Autodesk Inventor part; units mm, degrees
ref_plane "YZ Plane" through (0, 0, 0) normal (1, 0, 0) x (0, 1, 0)
ref_plane "XZ Plane" through (0, 0, 0) normal (0, 1, 0) x (-1, 0, 0)
ref_plane "XY Plane" through (0, 0, 0) normal (0, 0, 1) x (1, 0, 0)
sketch "Sketch1" plane through (0, 0, 0) normal (0, 0, 1) x (1, 0, 0)
  line L0 (-9.2194, -2.0534) -> (-9.2194, -17.5534)
  line L1 (-9.2194, -17.5534) -> (-15.6194, -17.5534)
  line L2 (-15.6194, -17.5534) -> (-15.6194, -2.0534)
  line L3 (-15.6194, -2.0534) -> (-9.2194, -2.0534)
  line L4 (-9.2194, 19.4466) -> (-9.2194, 3.9466)
  line L5 (-9.2194, 3.9466) -> (-15.6194, 3.9466)
  line L6 (-15.6194, 3.9466) -> (-15.6194, 19.4466)
  line L7 (-15.6194, 19.4466) -> (-9.2194, 19.4466)
  line L8 (14.7806, 19.4466) -> (14.7806, 3.9466)
  line L9 (14.7806, 3.9466) -> (8.3806, 3.9466)
  line L10 (8.3806, 3.9466) -> (8.3806, 19.4466)
  line L11 (8.3806, 19.4466) -> (14.7806, 19.4466)
  line L12 (14.7806, -1.568) -> (14.7806, -17.068)
  line L13 (14.7806, -17.068) -> (8.3806, -17.068)
  line L14 (8.3806, -17.068) -> (8.3806, -1.568)
  line L15 (8.3806, -1.568) -> (14.7806, -1.568)
  line L16 (20.7806, -27.5534) -> (20.7806, 25.4466)
  line L17 (20.7806, 25.4466) -> (-21.6194, 25.4466)
  line L18 (-21.6194, 25.4466) -> (-21.6194, -27.5534)
  line L19 (-21.6194, -27.5534) -> (20.7806, -27.5534)
  circle A0 centre (-0.4194, 11.6966) radius 1.5
  circle A1 centre (-0.4194, -9.8034) radius 1.5
  point P0 (0, 0)
extrude "Extrusion1" add sketch "Sketch1" along normal blind 6
properties part number "spoolHolderHolder"
Geometry: final body of the model. Coordinates: model frame, mm. A direction names the side the tool comes from. Round coordinates to 2 decimals unless told otherwise and drop trailing zeros. Order: outer loops, then holes, each group sorted by start corner. A loop starts at its lowest first (then second) coordinate and runs counter-clockwise, first axis right, second up. Notation, with made-up numbers: M 14,23 L 18,23 A18 ccw 18,51 Z; hole C 76.5,45 d5. An arc over 180 degrees is marked long. Use one line per item in the form item = value. Start each with the question number.
Q1. Access query for faces 4 (the face through (-9.219, 12, 3)), 5 (the face through (-1, -1, 0)). Directions: +Z, -Z, +X, -X, +Y, -Y. A direction counts if a zero-diameter tool reaches every point of the face in a straight line with its end or side. Return the directions, or none.
Q2. Cut plane B-B (y = -14.5). Return loops of the section in (x, z).
Q3. Mould query, pull axis Y, two halves, no side actions, for faces 1 (the face through (-1, -27.553, 3)), 2 (the face through (-1, -1, 6)), 3 (the face through (-15.619, 12, 3)). Classes: +Y half, -Y half, draft (parallel to the pull), parting line (faces both ways), or undercut.
Q4. Cut plane C-C (z = 0.55). Return loops of the section in (x, y).
Q5. Material intervals for line 1 (Y direction, x = -12, z = 4.2); line 2 (Y direction, x = 9, z = 3.5); line 3 (X direction, y = 9, z = 0.85), sorted ascending. Write a range as [from, to].
Q6. Pin query (flat end, axial travel): pin 1 Ø2.5 at (x, y) = (-0.42, 11.7) entering from +Z. Return the tip coordinate at first contact, or that it passes through.
Q7. Cut plane A-A (x = 13). Return loops of the section in (y, z).
Geometry results:
q1.face_4 = +Z, -Z
q1.face_5 = -Z, +X, -X, +Y, -Y
q2.outline = M -21.62,0 L -15.62,0 L -15.62,6 L -21.62,6 Z; M -9.22,0 L 8.38,0 L 8.38,6 L -9.22,6 Z; M 14.78,0 L 20.78,0 L 20.78,6 L 14.78,6 Z
q3.face_1 = -Y half
q3.face_2 = draft
q3.face_3 = undercut
q4.outline = M -21.62,-27.55 L 20.78,-27.55 L 20.78,25.45 L -21.62,25.45 Z; hole M -15.62,-17.55 L -9.22,-17.55 L -9.22,-2.05 L -15.62,-2.05 Z; hole M -15.62,3.95 L -9.22,3.95 L -9.22,19.45 L -15.62,19.45 Z; hole C -0.42,-9.8 d3; hole C -0.42,11.7 d3; hole M 8.38,-17.07 L 14.78,-17.07 L 14.78,-1.57 L 8.38,-1.57 Z; hole M 8.38,3.95 L 14.78,3.95 L 14.78,19.45 L 8.38,19.45 Z
q5.line_1 = [-27.55, -17.55], [-2.05, 3.95], [19.45, 25.45]
q5.line_2 = [-27.55, -17.07], [-1.57, 3.95], [19.45, 25.45]
q5.line_3 = [-21.62, -15.62], [-9.22, 8.38], [14.78, 20.78]
q6.pin_1 = through
q7.outline = M -27.55,0 L -17.07,0 L -17.07,6 L -27.55,6 Z; M -1.57,0 L 3.95,0 L 3.95,6 L -1.57,6 Z; M 19.45,0 L 25.45,0 L 25.45,6 L 19.45,6 Z
